Can you work these out from the model? Positions are in its coordinate system, mm. A direction names the side the tool comes from. Coordinates: 2 decimals unless noted, no trailing zeros. Write each loop counter-clockwise with the first axis right and the second up, starting at its lowest first coordinate (ties: lowest second). Pieces come first, ordered by that corner, then holes. Notation, with made-up numbers: (-29.5, 75) - (16.5, 75) arc R26 cw to (16.5, 98) - close; hole circle Ø9 at (33.25, 52). An arc over 180 degrees is marked (long way). Use one line per item in the form item = value. Start each with the question number.
(1) Thinking about a two-plate mould opening in X: for faces 3 (the face through (80, -71, 7)), 4 (the face through (389.66, -24.71, 7.4)), 5 (the face through (332.35, -37.42, 7.4)), 6 (the face through (410, -26, 7)), which applies, pulls with the +X half, pulls with the -X half, needs draft (parallel to the pull), parting line crosses it, or undercut?
(2) If we section it at B-B on x = 295: Please give me the cut outline in (y, z).
(3) For pin 1 Ø2 at (x, y) = (155.5, -48) entering from -Z; pin 2 Ø4 at (x, z) = (153.5, 9) entering from -Y; pin 3 Ø5 at (x, z) = (140.5, 11) entering from -Y; pin 4 Ø7.5 at (x, z) = (45.5, 8.5) entering from -Y, each with a flat end and sliding along its axis, tell me the tip position at first contact or that it passes through.
(4) If we section it at C-C on y = -57: Please give me the cut outline in (x, z), then the cut area to 3 significant figures.
(5) If we section it at A-A on z = 9: Please give me the cut outline in (x, y).
(6) On a 3-axis mill with a long thin cutter (end or side, diameter ignored), from which of +Z, -Z, +X, -X, +Y, -Y can I reach the whole of each face in a straight line? I mean faces 1 (the face through (41, -30, 7)), 2 (the face through (406.99, -2.85, 7.6)). Say none if no direction works.
(7) If we section it at D-D on x = 27: Please give me the cut outline in (y, z).
(8) If I drill on probe 1 along X at (y, z) = (-40, 2.5); probe 2 along X at (y, z) = (-35, 11.5); probe 3 along X at (y, z) = (-44, 2), over which ranges is the centre line in solid material (lowest first)? Write a range as from..to.
```python
from build123d import *

# Parameters (mm, degrees)
ESQUISSE1_R        = 10
BOSS_EXTRU_1_DEPTH = 15
CONG_1_R           = 10


with BuildPart() as part:
    # Esquisse1 → Boss.-Extru.1 (new body)
    with BuildSketch(Plane.XY):
        Polygon((0, 0), (410, 0), (410, -50), (80, -110), (80, -30), (0, -30), align=None)
        with Locations((300.451747289, -34.958932065)):
            Circle(ESQUISSE1_R, mode=Mode.SUBTRACT)
        with Locations((340.287475547, -31.337502223)):
            Circle(ESQUISSE1_R, mode=Mode.SUBTRACT)
        with Locations((380.123203806, -27.716072381)):
            Circle(ESQUISSE1_R, mode=Mode.SUBTRACT)
    extrude(amount=BOSS_EXTRU_1_DEPTH)

    # Congé1
    cong_1_edges = [part.edges().sort_by_distance(p)[0] for p in [
        (0, 0, 7.5),
        (410, 0, 7.5),
        (410, -50, 7.5),
    ]]
    fillet(cong_1_edges, radius=CONG_1_R)


solid = part.part
```
Reported:
q1.face_3 = pulls with the -X half
q1.face_4 = undercut
q1.face_5 = undercut
q1.face_6 = pulls with the +X half
q2.outline = (-70.91, 0) - (-43.34, 0) - (-43.34, 15) - (-70.91, 15) - close; (-26.58, 0) - (0, 0) - (0, 15) - (-26.58, 15) - close
q3.pin_1 = 0
q3.pin_2 = -97
q3.pin_3 = -99.45
q3.pin_4 = -30
q4.outline = (80, 0) - (371.5, 0) - (371.5, 15) - (80, 15) - close
q4.area = 4,370 mm2
q5.outline = (0, -30) - (80, -30) - (80, -110) - (401.79, -51.49) arc R10 ccw to (410, -41.65) - (410, -10) arc R10 ccw to (400, 0) - (10, 0) arc R10 ccw to (0, -10) - close; hole circle Ø20 at (300.45, -34.96); hole circle Ø20 at (340.29, -31.34); hole circle Ø20 at (380.12, -27.72)
q6.face_1 = +Z, -Z, -X, -Y
q6.face_2 = +Z, -Z, +X, +Y
q7.outline = (-30, 0) - (0, 0) - (0, 15) - (-30, 15) - close
q8.probe_1 = 80..291.82, 309.09..335.29, 345.28..410
q8.probe_2 = 80..290.45, 310.45..330.98, 349.59..373.27, 386.97..410
q8.probe_3 = 80..296.18, 304.72..409.72
